from build123d import *

# Parameters (mm, degrees)
SKETCH_1_R           = 1.5
EXTRUDE_1_DEPTH      = 7
EXTRUDE_2_DEPTH      = 6
EXTRUDE_2_DEPTH_BACK = 1
SKETCH_1_4_R         = 1.5


with BuildPart() as part:
    # Sketch 1 → Extrude 1 (new body)
    with BuildSketch(Plane(origin=(0, 0, 0), x_dir=(1, 0, 0), z_dir=(0, 1, 0))):
        Polygon((2.713546265, 0), (1.356773133, 2.35), (-1.356773133, 2.35), (-2.713546265, 0), (-1.356773133, -2.35), (1.356773133, -2.35), align=None)
        with Locations(Location((0, 0, 0), (0, 0, 270))):
            Circle(SKETCH_1_R, mode=Mode.SUBTRACT)
    extrude(amount=-EXTRUDE_1_DEPTH)

    # Sketch 1_4 → Extrude 2 (add, two sides: drawn at the far end of the back side and taken through both)
    with BuildSketch(Plane(origin=(0, 0, 0), x_dir=(1, 0, 0), z_dir=(0, 1, 0)).offset(-EXTRUDE_2_DEPTH_BACK)):
        with Locations(Location((0, 0, 0), (0, 0, 270))):
            Circle(SKETCH_1_4_R)
    extrude(amount=EXTRUDE_2_DEPTH + EXTRUDE_2_DEPTH_BACK)


solid = part.part
Model file for the job. Use its own axes, mm. A direction names the side the tool comes from. Give positions to 0.01 mm unless a question says otherwise; leave off trailing zeros. Loops run counter-clockwise (first coordinate to the right, second up) from the corner with the lowest first, then second, coordinate; pieces in that order, holes last.
1) Flat gauge pin, fed straight in: pin 1 Ø1.5 at (x, z) = (0, -0.5) entering from -Y. Where does the tip first touch, or does it go through?
2) Saw through at C-C (x = -0.5). Write the cut outline in (y, z), plus the area to 3 significant figures.
3) Saw through at A-A (y = -2.25). Write the cut outline in (x, z), plus the area to 3 significant figures.
4) Saw through at D-D (y = 3.75). Write the cut outline in (x, z), plus the area to 3 significant figures.
5) Pull direction Z, two halves, no side cores. Call faces 1 (the flat face through (2.026, -3.451, 1.191)), 2 (the flat face through (-2.026, -3.451, -1.191)), 3 (the flat face through (0, -1, 0)): +Z half, -Z half, draft (parallel to the pull), parting line (faces both ways), or undercut.
6) Saw through at B-B (z = 0.95). Write the cut outline in (x, y), plus the area to 3 significant figures.
7) Tool access for faces 4 (the flat face through (-2.045, -3.451, 1.159)), 5 (the cylindrical face through (0.45, -3.96, 1.43)), 6 (the cylindrical face through (0.45, 2.96, 1.43)): list every direction of +Z, -Z, +X, -X, +Y, -Y with a clear straight run to the whole face (end or side of a thin tool).
8) Wall check: line 1 (Y direction, x = -1.25, z = -0.6); line 2 (X direction, y = -1.25, z = 1.2); line 3 (Z direction, x = 0.1, y = 1.25). Give the ranges that are in metal, low to high.
Answer block:
1. pin 1: stops at y = -1
2. outline: (-7, -2.35) - (0, -2.35) - (0, -1.41) - (6, -1.41) - (6, 1.41) - (0, 1.41) - (0, 2.35) - (-7, 2.35) - (-7, 1.41) - (-1, 1.41) - (-1, -1.41) - (-7, -1.41) - close
2. area: 32.9 mm2
3. outline: (-2.71, 0) - (-1.36, -2.35) - (1.36, -2.35) - (2.71, 0) - (1.36, 2.35) - (-1.36, 2.35) - close; hole circle Ø3 at (0, 0)
3. area: 12.1 mm2
4. outline: circle Ø3 at (0, 0)
4. area: 7.07 mm2
5. face 1: +Z half
5. face 2: -Z half
5. face 3: undercut
6. outline: (-2.17, -7) - (-1.16, -7) - (-1.16, -1) - (1.16, -1) - (1.16, -7) - (2.17, -7) - (2.17, 0) - (1.16, 0) - (1.16, 6) - (-1.16, 6) - (-1.16, 0) - (-2.17, 0) - close
6. area: 30.3 mm2
7. face 4: +Z, -X, +Y, -Y
7. face 5: -Y
7. face 6: +Y
8. line 1: y = -1 to 6
8. line 2: x = -2.02 to -0.9, 0.9 to 2.02
8. line 3: z = -1.5 to 1.5
